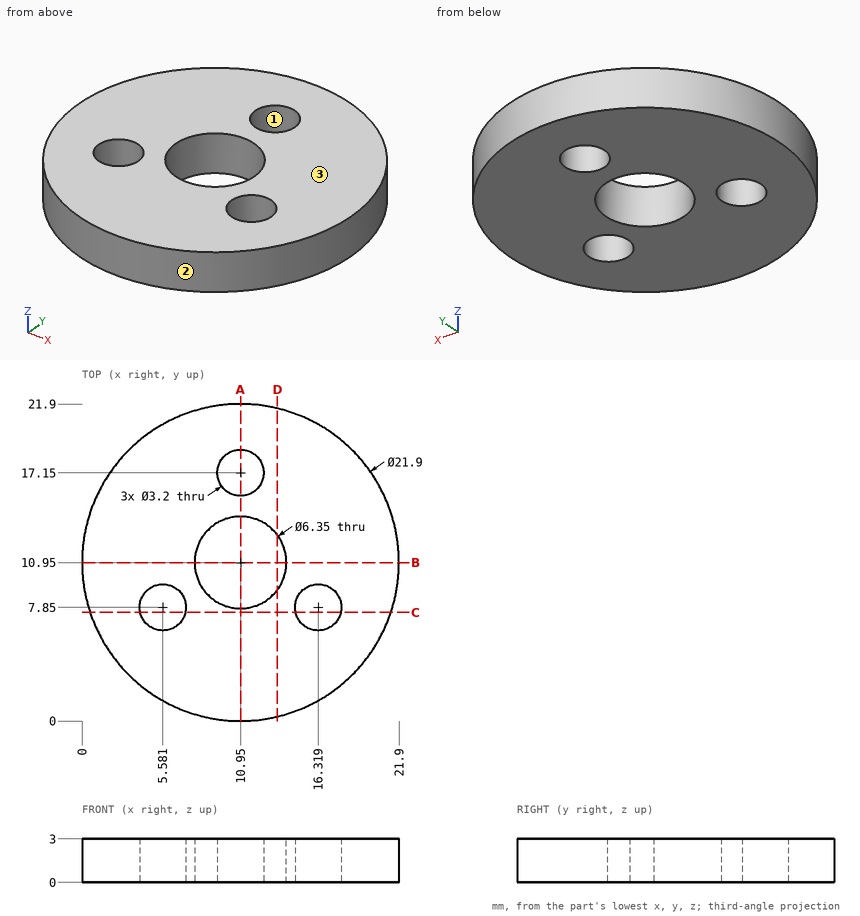
Verification items for this drawing (mm, ordinates from the low corner). Round coordinates to 2 decimals unless told otherwise and drop trailing zeros. Order: outer loops, then holes, each group sorted by start corner. A loop starts at its lowest first (then second) coordinate and runs counter-clockwise, first axis right, second up.
1) Depth check by flat-ended pin: pin 1 (1.5 mm diameter, centred on y = 14.5, z = 2.5, fed in from -X); pin 2 (1.9 mm diameter, centred on x = 5.58, y = 7.85, fed in from -Z). Enter the tip coordinate at first touch or a pass-through.
Geometry says:
pin 1: stops at x = 0.36
pin 2: passes through
2) Cross-section at A-A, the plane x = 10.95. Give the number of separate pieces and of enclosed holes in the cut face.
Geometry says:
separate pieces: 3
enclosed holes: 0
3) Draft check along X on the marked faces 1, 2 and 3. Enter one of: +X half, -X half, draft (parallel to the pull), parting line (faces both ways), or undercut.
Geometry says:
face 1: undercut
face 2: parting line
face 3: draft
4) Material ranges on line 1 (Y direction, x = 11, z = 0.75) (1 decimal); line 2 (Y direction, x = 2.5, z = 0.2) (1 decimal); line 3 (Y direction, x = 6.25, z = 1.8), recorded low to high.
Geometry says:
line 1: y = 0 to 7.8, 14.1 to 15.6, 18.7 to 21.9
line 2: y = 4 to 17.9
line 3: y = 1.06 to 6.4, 9.3 to 20.84
5) Cross-section at D-D, the plane x = 13.5. Record the cut outline in (y, z).
Geometry says:
outline: (0.3, 0) - (9.06, 0) - (9.06, 3) - (0.3, 3) - close; (12.84, 0) - (21.6, 0) - (21.6, 3) - (12.84, 3) - close
6) Cross-section at C-C, the plane y = 7.5. Record the cut outline in (x, z).
Geometry says:
outline: (0.56, 0) - (4.02, 0) - (4.02, 3) - (0.56, 3) - close; (7.14, 0) - (14.76, 0) - (14.76, 3) - (7.14, 3) - close; (17.88, 0) - (21.34, 0) - (21.34, 3) - (17.88, 3) - close
7) Cross-section at B-B, the plane y = 10.95. Record the cut outline in (x, z) (1 decimal).
Geometry says:
outline: (0, 0) - (7.8, 0) - (7.8, 3) - (0, 3) - close; (14.1, 0) - (21.9, 0) - (21.9, 3) - (14.1, 3) - close
